Answer from the drawing. Dimensions are ordinates in mm from the lowest x, y and z of the part. A direction names the side the tool comes from. Give positions to 0.01 mm unless a question says otherwise; leave off trailing zeros. Loops run counter-clockwise (first coordinate to the right, second up) from the corner with the lowest first, then second, coordinate; pieces in that order, holes last. Notation, with made-up numbers: (-27, 10) -> (-20, 10) arc R26 cw to (-20, 31) -> close; hole circle Ø9 at (11.25, 82.5). An arc over 180 degrees is marked (long way). Write each question's results on one line, items separated by ' | '. Start each with the question number.
Item 1: Each of these flat-tipped pins is pushed along its axis until it touches: P1, Ø2.5, axis at x = 23.876, y = 25.4, coming from the +Z side (1 decimal); P2, Ø6.5, axis at x = 16, z = 7.5, coming from the +Y side (1 decimal). Where does it stop, or does it pass through?
Item 2: Which of the six approach directions +Z, -Z, +X, -X, +Y, -Y give full straight-line access (tool end or side, diameter ignored) to the marked faces 1 and 2?
Item 3: Section D-D on x = 12.5 is taken. Write down the section's boundary in (y, z) (1 decimal), and give its area (3 significant figures).
Item 4: Determine the mould class of the marked faces 3, 4 and 5 for opening direction Y: +Y half, -Y half, draft (parallel to the pull), parting line (faces both ways), or undercut.
Item 5: Find the intervals of material crossed by line 1 (Z direction, x = 9.5, y = 14) (1 decimal); line 2 (Y direction, x = 24.5, z = 2.75) (1 decimal), in increasing order.
Item 6: Section A-A on x = 25.4 is taken. Write down the section's boundary in (y, z) (1 decimal).
Item 7: Section B-B on z = 8.5 is taken. State how many separate pieces and enclosed holes the cut face has.
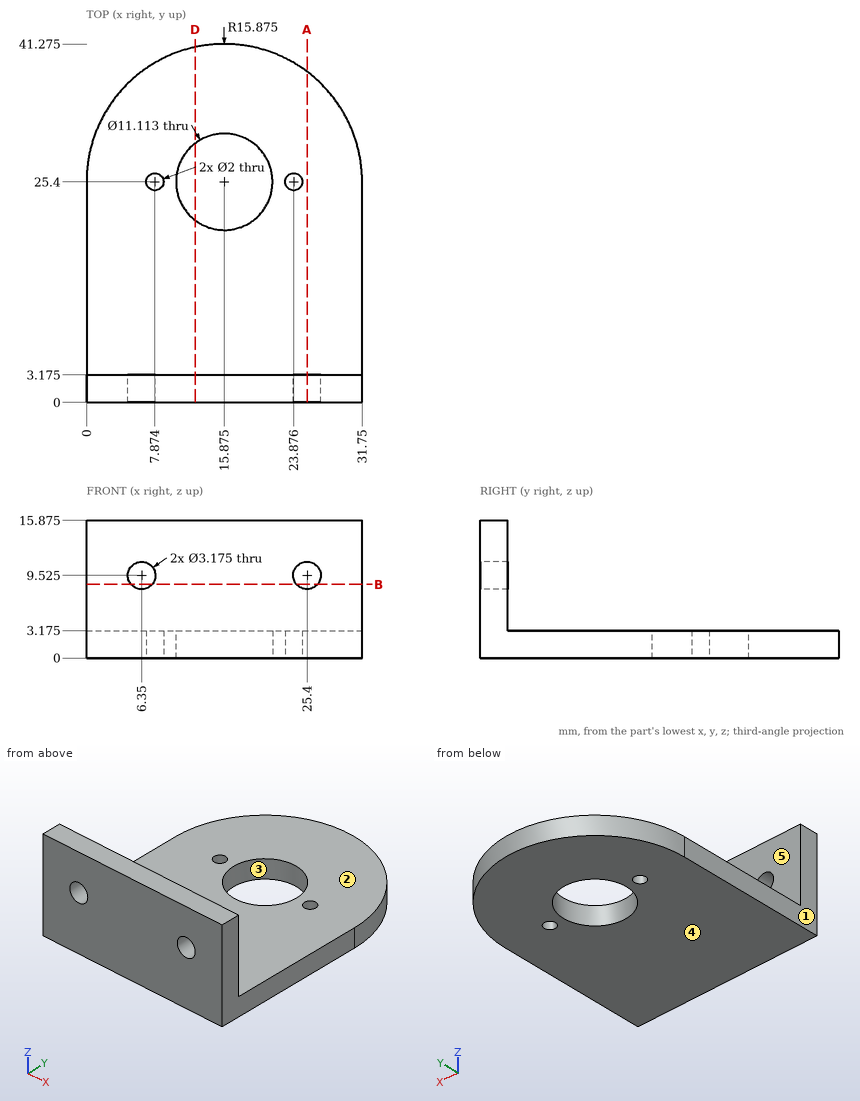
Findings:
1) P1: z = 3.2 | P2: y = 3.2
2) face 1: +Z, -Z, -X, +Y, -Y | face 2: +Z, +X, -X, +Y
3) outline: (0, 0) -> (21, 0) -> (21, 3.2) -> (3.2, 3.2) -> (3.2, 15.9) -> (0, 15.9) -> close; (29.8, 0) -> (40.9, 0) -> (40.9, 3.2) -> (29.8, 3.2) -> close | area: 142 mm2
4) face 3: undercut | face 4: draft | face 5: +Y half
5) line 1: 0 to 3.2 | line 2: 0 to 24.6, 26.2 to 38.7
6) outline: (0, 0) -> (38.1, 0) -> (38.1, 3.2) -> (3.2, 3.2) -> (3.2, 7.9) -> (0, 7.9) -> close; (0, 11.1) -> (3.2, 11.1) -> (3.2, 15.9) -> (0, 15.9) -> close
7) separate pieces: 3 | enclosed holes: 0
